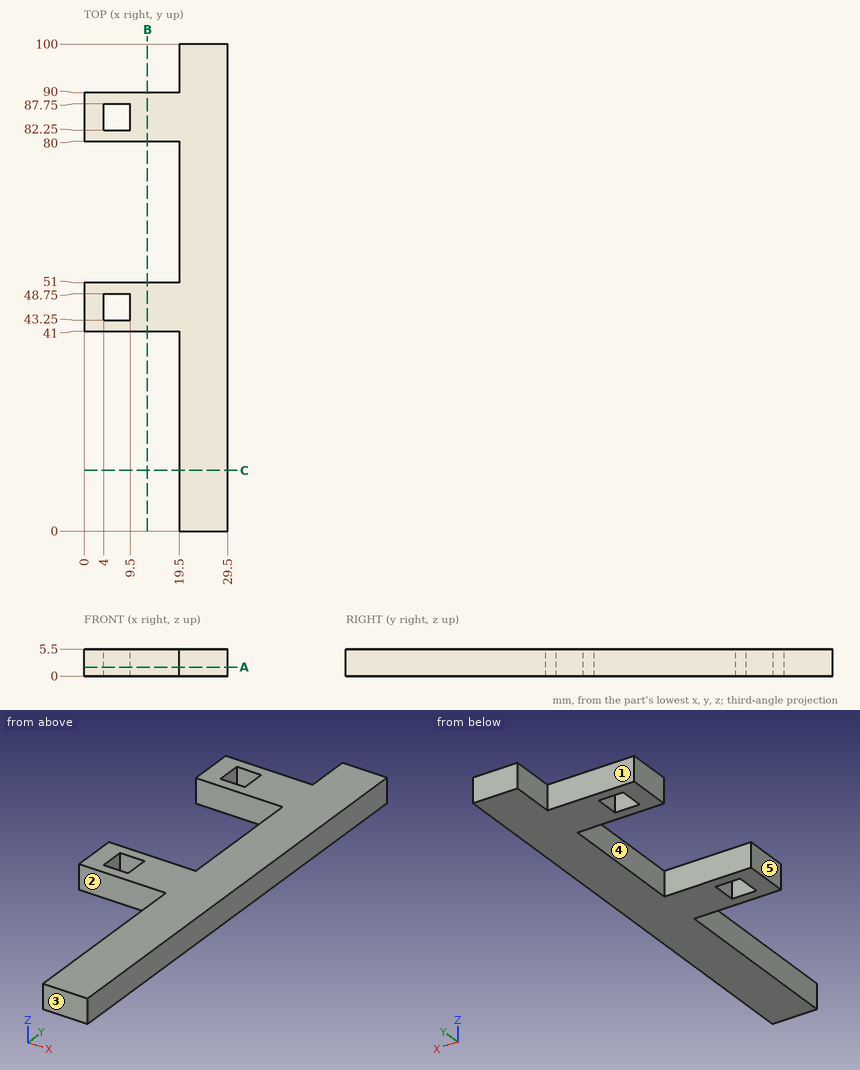
The drawing under review shows one solid part. Ordinate dimensions are in mm from its lowest x, y, z. A direction names the side the tool comes from. Round coordinates to 2 decimals unless told otherwise and drop trailing zeros. Order: outer loops, then holes, each group sorted by start corner. A loop starts at its lowest first (then second) coordinate and runs counter-clockwise, first axis right, second up. Notation, with made-up numbers: (23.25, 36.5) -> (35.25, 36.5) arc R22 ccw to (35.25, 49.5) -> close; hole circle Ø7 at (4, -27.5). An arc over 180 degrees is marked (long way). Use a Markdown table: item, result.
Item 1: Take a section at C-C (y = 12.5). State the section outline as (x, z) points.
Resolved:
| item | result |
|---|---|
| outline | (19.5, 0) -> (29.5, 0) -> (29.5, 5.5) -> (19.5, 5.5) -> close |
Item 2: Take a section at B-B (x = 13). State the section outline as (y, z) points.
Resolved:
| item | result |
|---|---|
| outline | (41, 0) -> (51, 0) -> (51, 5.5) -> (41, 5.5) -> close; (80, 0) -> (90, 0) -> (90, 5.5) -> (80, 5.5) -> close |
Item 3: Machinability: for the marked faces 1, 2, 3, 4 and 5, which of the approach directions +Z, -Z, +X, -X, +Y, -Y give a long, thin tool a straight path to every point of the face, cutting with its end or side? Answer none if there is none.
Resolved:
| item | result |
|---|---|
| face 1 | +Z, -Z, -X, +Y |
| face 2 | +Z, -Z, -X, -Y |
| face 3 | +Z, -Z, +X, -X, -Y |
| face 4 | +Z, -Z, -X |
| face 5 | +Z, -Z, -X, +Y, -Y |
Item 4: Take a section at A-A (z = 1.8). State the section outline as (x, y) points, plus the area to 3 significant figures.
Resolved:
| item | result |
|---|---|
| outline | (0, 41) -> (19.5, 41) -> (19.5, 0) -> (29.5, 0) -> (29.5, 100) -> (19.5, 100) -> (19.5, 90) -> (0, 90) -> (0, 80) -> (19.5, 80) -> (19.5, 51) -> (0, 51) -> close; hole (4, 43.25) -> (9.5, 43.25) -> (9.5, 48.75) -> (4, 48.75) -> close; hole (4, 82.25) -> (9.5, 82.25) -> (9.5, 87.75) -> (4, 87.75) -> close |
| area | 1,330 mm² |
Item 5: For pin 1 (10 mm diameter, centred on x = 25.5, y = 88, fed in from -Z); pin 2 (1 mm diameter, centred on x = 8, z = 5, fed in from -Y); pin 3 (3 mm diameter, centred on y = 71.5, z = 3.5, fed in from -X), all flat-tipped, find the tip position at first contact; note any pin that passes through.
Resolved:
| item | result |
|---|---|
| pin 1 | stops at z = 0 |
| pin 2 | stops at y = 41 |
| pin 3 | stops at x = 19.5 |
Item 6: For line 1 along Y through (x, z) = (6.5, 0.75); line 2 along Y through (x, z) = (15.5, 2.8); line 3 along X through (y, z) = (48, 5.05), list the stretches that pass through material, from the lowest coordinate up. Write a range as [from, to].
Resolved:
| item | result |
|---|---|
| line 1 | y = [41, 43.25], [48.75, 51], [80, 82.25], [87.75, 90] |
| line 2 | y = [41, 51], [80, 90] |
| line 3 | x = [0, 4], [9.5, 29.5] |
